```python
from build123d import *

# Parameters (mm, degrees)
EXTRUDE_1_DEPTH     = 4
SKETCH_2_W          = 4
SKETCH_2_H          = 20
EXTRUDE_2_DEPTH     = 5
SKETCH_3_W          = 5
SKETCH_3_H          = 4.35
CUT_EXTRUDE_1_DEPTH = 4
SKETCH_4_R          = 1.25
CUT_EXTRUDE_2_DEPTH = 11.3
SKETCH_6_R          = 5
CUT_EXTRUDE_4_DEPTH = 2


with BuildPart() as part:
    # 草图1 → 凸台-拉伸1 (new body)
    with BuildSketch(Plane.XY):
        with BuildLine():
            Line((0, 10), (37, 10))
            ThreePointArc((37, 10), (47, 0), (37, -10))
            Line((37, -10), (0, -10))
            Line((0, -10), (-10, -10))
            Line((-10, -10), (-10, 10))
            Line((-10, 10), (0, 10))
        make_face()
    extrude(amount=EXTRUDE_1_DEPTH)

    # 草图2 → 凸台-拉伸2 (add)
    with BuildSketch(Plane.ZY.offset(10)):
        with Locations((2, 0)):
            Rectangle(SKETCH_2_W, SKETCH_2_H)
    extrude(amount=EXTRUDE_2_DEPTH)

    # 草图3 → 切除-拉伸1 (cut)
    with BuildSketch(Plane.XY.offset(4)):
        with Locations((-12.5, 7.825)):
            Rectangle(SKETCH_3_W, SKETCH_3_H)
        with Locations((-12.5, -7.825)):
            Rectangle(SKETCH_3_W, SKETCH_3_H)
    extrude(amount=-CUT_EXTRUDE_1_DEPTH, mode=Mode.SUBTRACT)

    # 草图4 → 切除-拉伸2 (cut)
    with BuildSketch(Plane(origin=(0, 5.65, 0), x_dir=(1, 0, 0), z_dir=(0, 1, 0))):
        with Locations(Location((-12.379659001, -2, 0), (0, 0, 270))):
            Circle(SKETCH_4_R)
    extrude(amount=-CUT_EXTRUDE_2_DEPTH, mode=Mode.SUBTRACT)

    # 草图6 → 切除-拉伸4 (cut)
    with BuildSketch(Plane.XY.offset(4)):
        with Locations((37, 0)):
            Circle(SKETCH_6_R)
        with Locations((2, 0)):
            Circle(SKETCH_6_R)
    extrude(amount=-CUT_EXTRUDE_4_DEPTH, mode=Mode.SUBTRACT)


solid = part.part
```
The model under review builds one solid part; all positions refer to its coordinate system, in mm. A direction names the side the tool comes from. Round coordinates to 2 decimals unless told otherwise and drop trailing zeros. Write each loop counter-clockwise with the first axis right and the second up, starting at its lowest first coordinate (ties: lowest second). Pieces come first, ordered by that corner, then holes. Notation, with made-up numbers: (0.5, 60.25) - (45.5, 60.25) arc R15 ccw to (45.5, 87.25) - close; hole circle Ø10 at (67, 66). An arc over 180 degrees is marked (long way). Answer as CSV lines item,"result". Start each with the question number.
(1) We need section D-D on y = 3. State the section outline as (x, z) points, plus the area to 3 significant figures.
(2) We need section A-A on x = 2. State the section outline as (y, z) points.
(3) To check wall thickness, follow line 1 (Y direction, x = 2, z = 3.3); line 2 (X direction, y = -5.25, z = 2.75); line 3 (X direction, y = -3.25, z = 2.35). State the ranges of each line that lie inside material, in increasing order.
(4) For faces 1 (the flat face through (16, 0, 4)), 2 (the cylindrical face through (6.619, -1.915, 3.014)), 3 (the flat face through (-14, 5.65, 2)), 4 (the flat face through (-10, -8, 2)), list the 3-axis set-ups (+Z, -Z, +X, -X, +Y, -Y) from which the entire face can be reached by the end or side of a thin tool; tool diameter is ignored.
(5) For pin 1 Ø2 at (y, z) = (-7, 2) entering from -X; pin 2 Ø2 at (y, z) = (-7, 1) entering from +X; pin 3 Ø1 at (y, z) = (-1.5, 1.5) entering from +X; pin 4 Ø2 at (x, z) = (-12.38, 2) entering from -Y, all flat-tipped, find the tip position at first contact; note any pin that passes through.
(6) We need section B-B on y = 0. State the section outline as (x, z) points, plus the area to 3 significant figures.
(7) We need section C-C on x = 36. State the section outline as (y, z) points.
(8) Draft analysis for pull direction Y (two halves, no side actions). For faces 5 (the cylindrical face through (47, 0, 2)), 6 (the flat face through (14, -10, 2)), 7 (the flat face through (16, 0, 0)), 8 (the flat face through (2, 0, 2)), state which applies: pulls with the +Y half, pulls with the -Y half, needs draft (parallel to the pull), parting line crosses it, or undercut.
Worked answers:
1,outline,"(-15, 0) - (46.54, 0) - (46.54, 4) - (41, 4) - (41, 2) - (33, 2) - (33, 4) - (6, 4) - (6, 2) - (-2, 2) - (-2, 4) - (-15, 4) - close; hole circle Ø2.5 at (-12.38, 2)"
1,area,"209 mm²"
2,outline,"(-10, 0) - (10, 0) - (10, 4) - (5, 4) - (5, 2) - (-5, 2) - (-5, 4) - (-10, 4) - close"
3,line 1,"-10 to -5, 5 to 10"
3,line 2,"-15 to -13.38, -11.38 to 45.51"
3,line 3,"-15 to -13.58, -11.18 to -1.8, 5.8 to 33.2, 40.8 to 46.46"
4,face 1,"+Z, +X, -X, +Y, -Y"
4,face 2,"+Z"
4,face 3,"+Z, -Z, -X, +Y"
4,face 4,"+Z, -Z, -X, -Y"
5,pin 1,"x = -10"
5,pin 2,"x = 45"
5,pin 3,"x = 46.95"
5,pin 4,"through"
6,outline,"(-15, 0) - (47, 0) - (47, 4) - (42, 4) - (42, 2) - (32, 2) - (32, 4) - (7, 4) - (7, 2) - (-3, 2) - (-3, 4) - (-15, 4) - close; hole circle Ø2.5 at (-12.38, 2)"
6,area,"203 mm²"
7,outline,"(-10, 0) - (10, 0) - (10, 4) - (4.9, 4) - (4.9, 2) - (-4.9, 2) - (-4.9, 4) - (-10, 4) - close"
8,face 5,"parting line crosses it"
8,face 6,"pulls with the -Y half"
8,face 7,"needs draft"
8,face 8,"undercut"
